```python
from build123d import *

# Parameters (mm, degrees)
BASES_W                                         = 21.5
BASES_H                                         = 34.5
BASE_DEPTH                                      = 1.6
CSK_FOR_M3_FLAT_HEAD_MACHINE_SCREW1_D           = 3.4
CSK_FOR_M3_FLAT_HEAD_MACHINE_SCREW1_DEPTH       = 11
CSK_FOR_M3_FLAT_HEAD_MACHINE_SCREW1_CSINK_D     = 6.3
CSK_FOR_M3_FLAT_HEAD_MACHINE_SCREW1_CSINK_ANGLE = 90
CSK_FOR_M3_FLAT_HEAD_MACHINE_SCREW1_TIP         = 1.021463052
BORES_R                                         = 4.5
BORE_DEPTH                                      = 21.388354519
LOCKINGFEATURES_R                               = 1.1
LOCKING_FEATURE_DEPTH                           = 0.3
LF_DOME_FACE_RADIUS                             = 1.1
LF_DOME_HEIGHT                                  = 0.2
LF_HM_COPY_1_FACE_RADIUS                        = 1.1
LF_HM_COPY_1_HEIGHT                             = 0.2
LFBOTTOMCUT_R                                   = 1.1
LF_BOTTOM_CUT_DEPTH                             = 0.3
BASE_FILLET_R                                   = 1


with BuildPart() as part:
    # BaseS → BASE (new body)
    with BuildSketch(Plane(origin=(0, 0, 0), x_dir=(1, 0, 0), z_dir=(0, 1, 0))):
        Rectangle(BASES_W, BASES_H)
    extrude(amount=-BASE_DEPTH)

    # CSK for M3 Flat Head Machine Screw1
    with Locations(Plane(origin=(0, 0, 0), x_dir=(1, 0, 0), z_dir=(0, 1, 0))):
        with Locations((-7, 14), (7, -14)):
            CounterSinkHole(CSK_FOR_M3_FLAT_HEAD_MACHINE_SCREW1_D / 2, CSK_FOR_M3_FLAT_HEAD_MACHINE_SCREW1_CSINK_D / 2, depth=CSK_FOR_M3_FLAT_HEAD_MACHINE_SCREW1_DEPTH, counter_sink_angle=CSK_FOR_M3_FLAT_HEAD_MACHINE_SCREW1_CSINK_ANGLE)
            with Locations((0, 0, -(CSK_FOR_M3_FLAT_HEAD_MACHINE_SCREW1_DEPTH + CSK_FOR_M3_FLAT_HEAD_MACHINE_SCREW1_TIP / 2))):  # 118° drill point
                Cone(0, CSK_FOR_M3_FLAT_HEAD_MACHINE_SCREW1_D / 2, CSK_FOR_M3_FLAT_HEAD_MACHINE_SCREW1_TIP, mode=Mode.SUBTRACT)

    # BoreS → BORE (cut, through all)
    with BuildSketch(Plane(origin=(0, 0, 0), x_dir=(1, 0, 0), z_dir=(0, 1, 0))):
        with Locations(Location((0, 0, 0), (0, 0, 270))):
            Circle(BORES_R)
    extrude(amount=-BORE_DEPTH, mode=Mode.SUBTRACT)

    # LockingFeatureS → LOCKING FEATURE (add)
    with BuildSketch(Plane(origin=(0, 0, 0), x_dir=(1, 0, 0), z_dir=(0, 1, 0))):
        with Locations(Location((-7, 0, 0), (0, 0, 270))):
            Circle(LOCKINGFEATURES_R)
    locking_feature = extrude(amount=LOCKING_FEATURE_DEPTH)

    # LF DOME: a dome of height H over a round flat face of radius A is a cap of a sphere of radius (A * A + H * H) / (2 * H)
    lf_dome_r = (LF_DOME_FACE_RADIUS * LF_DOME_FACE_RADIUS + LF_DOME_HEIGHT * LF_DOME_HEIGHT) / (2 * LF_DOME_HEIGHT)
    lf_dome_base = Plane((-7, 0.3, 0), z_dir=(0, 1, 0))
    with Locations(lf_dome_base.offset(LF_DOME_HEIGHT - lf_dome_r)):
        lf_dome_ball = Sphere(lf_dome_r, mode=Mode.PRIVATE)
    add(split(lf_dome_ball, bisect_by=lf_dome_base, keep=Keep.TOP, mode=Mode.PRIVATE))

    # LF HM: LOCKING FEATURE across plane
    add(locking_feature.mirror(Plane(origin=(0, 0, 0), x_dir=(0, 0, 1), z_dir=(1, 0, 0))))

    # LF HM copy 1: a dome of height H over a round flat face of radius A is a cap of a sphere of radius (A * A + H * H) / (2 * H)
    lf_hm_copy_1_r = (LF_HM_COPY_1_FACE_RADIUS * LF_HM_COPY_1_FACE_RADIUS + LF_HM_COPY_1_HEIGHT * LF_HM_COPY_1_HEIGHT) / (2 * LF_HM_COPY_1_HEIGHT)
    lf_hm_copy_1_base = Plane((7, 0.3, 0), z_dir=(0, 1, 0))
    with Locations(lf_hm_copy_1_base.offset(LF_HM_COPY_1_HEIGHT - lf_hm_copy_1_r)):
        lf_hm_copy_1_ball = Sphere(lf_hm_copy_1_r, mode=Mode.PRIVATE)
    add(split(lf_hm_copy_1_ball, bisect_by=lf_hm_copy_1_base, keep=Keep.TOP, mode=Mode.PRIVATE))

    # LFBottomCut → LF BOTTOM CUT (cut)
    with BuildSketch(Plane(origin=(0, -1.6, 0), x_dir=(-1, 0, 0), z_dir=(0, -1, 0))):
        with Locations(Location((7, 0, 0), (0, 0, 270))):
            Circle(LFBOTTOMCUT_R)
        with Locations(Location((-7, 0, 0), (0, 0, 270))):
            Circle(LFBOTTOMCUT_R)
    extrude(amount=-LF_BOTTOM_CUT_DEPTH, mode=Mode.SUBTRACT)

    # BASE FILLET
    base_fillet_edges = [part.edges().sort_by_distance(p)[0] for p in [
        (10.75, -0.8, 17.25),
        (-10.75, -0.8, 17.25),
        (-10.75, -0.8, -17.25),
        (10.75, -0.8, -17.25),
    ]]
    fillet(base_fillet_edges, radius=BASE_FILLET_R)


solid = part.part
```
Read the model definition and answer for the solid it produces. Units are mm, in the model's axes. A direction names the side the tool comes from. Round coordinates to 2 decimals unless told otherwise and drop trailing zeros. Write each loop counter-clockwise with the first axis right and the second up, starting at its lowest first coordinate (ties: lowest second). Pieces come first, ordered by that corner, then holes. Notation, with made-up numbers: M 77,-20.75 L 86,-20.75 A14 cw 86,-2.75 Z; hole C 14.25,63 d8. An arc over 180 degrees is marked long. One line per item, written item: value.
Q1. Straight lines are drawn through the part: line 1 (X direction, y = -1.5, z = 0); line 2 (X direction, y = -1, z = 0); line 3 (X direction, y = -1.5, z = -14). For each, find the intervals that lie inside material, in ascending order. Write a range as [from, to].
Data:
line 1: [-10.75, -8.1], [-5.9, -4.5], [4.5, 5.9], [8.1, 10.75]
line 2: [-10.75, -4.5], [4.5, 10.75]
line 3: [-10.75, -8.7], [-5.3, 10.75]
Q2. Which of the six approach directions +Z, -Z, +X, -X, +Y, -Y give full straight-line access (tool end or side, diameter ignored) to faces 5 (the cylindrical face through (-7.67, 0.15, -0.87)), 6 (the flat face through (0, -1, -17.25)), 7 (the flat face through (-7, -1.3, 0))?
Data:
face 5: +Y
face 6: -Z, +X, -X, +Y, -Y
face 7: -Y
Q3. Find section A-A on z = 14. Write down the section's boundary in (x, y).
Data:
outline: M -10.75,-1.6 L 5.3,-1.6 L 5.3,-1.45 L 3.85,0 L -10.75,0 Z; M 8.7,-1.6 L 10.75,-1.6 L 10.75,0 L 10.15,0 L 8.7,-1.45 Z
Q4. For a pull along X with two mould halves and no side action, classify faces 1 (the cylindrical face through (10.449, -0.811, 16.965)), 2 (the flat face through (0, -1, 17.25)), 3 (the cylindrical face through (-10.465, -0.811, -16.949)), 4 (the cylindrical face through (1.352, -0.789, 4.292)) as +X half, -X half, draft (parallel to the pull), parting line (faces both ways), or undercut.
Data:
face 1: +X half
face 2: draft
face 3: -X half
face 4: undercut
Q5. Find section B-B on x = 7. Write down the section's boundary in (y, z) (3 decimals).
Data:
outline: M -1.6,-17.25 L 0,-17.25 L 0,-1.1 L 0.3,-1.1 A3.125 ccw 0.3,1.1 L 0,1.1 L 0,10.85 L -1.45,12.3 L -1.6,12.3 L -1.6,1.1 L -1.3,1.1 L -1.3,-1.1 L -1.6,-1.1 Z; M -1.6,15.7 L -1.45,15.7 L 0,17.15 L 0,17.25 L -1.6,17.25 Z
Q6. Find section C-C on y = -0.6. Write down the section's boundary in (x, z).
Data:
outline: M -10.75,-16.25 A1 ccw -9.75,-17.25 L 9.75,-17.25 A1 ccw 10.75,-16.25 L 10.75,16.25 A1 ccw 9.75,17.25 L -9.75,17.25 A1 ccw -10.75,16.25 Z; hole C -7,-14 d5.1; hole C 0,0 d9; hole C 7,14 d5.1
Q7. Find section D-D on z = 0. Write down the section's boundary in (x, y) (3 decimals).
Data:
outline: M -10.75,-1.6 L -8.1,-1.6 L -8.1,-1.3 L -5.9,-1.3 L -5.9,-1.6 L -4.5,-1.6 L -4.5,0 L -5.9,0 L -5.9,0.3 A3.125 ccw -8.1,0.3 L -8.1,0 L -10.75,0 Z; M 4.5,-1.6 L 5.9,-1.6 L 5.9,-1.3 L 8.1,-1.3 L 8.1,-1.6 L 10.75,-1.6 L 10.75,0 L 8.1,0 L 8.1,0.3 A3.125 ccw 5.9,0.3 L 5.9,0 L 4.5,0 Z
Q8. Flat-ended cylindrical pins translate along their axes: pin 1 Ø2 at (x, z) = (7, 14) entering from +Y; pin 2 Ø0.7 at (x, z) = (-7.5, 0.5) entering from -Y; pin 3 Ø1.8 at (x, z) = (7, -0.5) entering from -Y. Find the tip coordinate at first contact, or state that the pin passes through.
Data:
pin 1: through
pin 2: y = -1.3
pin 3: y = -1.6
